Could you check a few things on this model? Use its own coordinates, in mm. A direction names the side the tool comes from. Coordinates: 2 decimals unless noted, no trailing zeros. Write each loop counter-clockwise with the first axis right and the second up, starting at its lowest first coordinate (ties: lowest second). Pieces come first, ordered by that corner, then holes.
Item 1: I want a section at A-A on x = 11. Please give me the cut outline in (y, z), then the cut area to 3 significant figures.
Item 2: I want a section at D-D on x = 23. Please give me the cut outline in (y, z).
Item 3: I want a section at B-B on y = -23. Please give me the cut outline in (x, z), then the cut area to 3 significant figures.
Item 4: Which directions (+Z, -Z, +X, -X, +Y, -Y) give clear straight access to the entire face, cutting with the end or side of a thin tool? Please do faces 4 (the cylindrical face through (-27.454, -13.85, 14.954)), 5 (the flat face through (34, 6, 15.5)), 6 (the flat face through (5, 4, 5.6)), 7 (the flat face through (23, -8, 25)).
Item 5: If I drill on probe 1 along Y at (x, z) = (27.5, 10.75); probe 2 along Y at (x, z) = (1, 19.5); probe 3 along Z at (x, y) = (5, 1), over which ranges is the centre line in solid material (lowest first)?
Item 6: For P1, Ø2, axis at y = 8.5, z = 21.5, coming from the -X side; P2, Ø4.5, axis at x = -30, z = 19.5, coming from the -Y side; P3, Ø0.6, axis at x = 29, z = 3, coming from the +Y side, each with a flat end and sliding along its axis, tell me the tip position at first contact or that it passes through.
Item 7: I want a section at C-C on y = -13.55. Please give me the cut outline in (x, z), then the cut area to 3 significant figures.
Item 8: Thinking about a two-plate mould opening in X: for faces 1 (the flat face through (29, -27.7, 4)), 2 (the flat face through (34, 6, 20.5)), 3 (the flat face through (30, -4, 20)), which applies, +X half, -X half, draft (parallel to the pull), parting line (faces both ways), or undercut?
from build123d import *

# Parameters (mm, degrees)
BOSS_EXTRUDE1_DEPTH = 25
SKETCH2_W           = 57.7
SKETCH2_H           = 16.5
CUT_EXTRUDE1_DEPTH  = 52.159456604
SKETCH3_W           = 30
SKETCH3_H           = 20
CUT_EXTRUDE2_DEPTH  = 7.5
CUT_EXTRUDE3_REACH  = 58.541
SKETCH4_R           = 2
SKETCH5_R           = 2
CUT_EXTRUDE4_DEPTH  = 1.5
SKETCH6_W           = 7
SKETCH6_H           = 8
BOSS_EXTRUDE2_DEPTH = 2
SKETCH7_W           = 4
SKETCH7_H           = 20.2
BOSS_EXTRUDE3_DEPTH = 2
BOSS_EXTRUDE4_DEPTH = 7
SKETCH9_W           = 32
SKETCH9_H           = 22
CUT_EXTRUDE5_DEPTH  = 2
FILLET1_R           = 1
FILLET2_R           = 1
SKETCH10_R          = 1
BOSS_EXTRUDE5_DEPTH = 1.5
FILLET3_R           = 1
BOSS_EXTRUDE6_DEPTH = 2.7
CUT_EXTRUDE6_REACH  = 82.092
SKETCH13_W          = 4.5
SKETCH13_H          = 8.8
BOSS_EXTRUDE7_DEPTH = 2
SKETCH14_W          = 10
SKETCH14_H          = 3.4
CUT_EXTRUDE7_DEPTH  = 54.232805215
SKETCH15_R          = 1.55
CUT_EXTRUDE8_DEPTH  = 2.5


with BuildPart() as part:
    # Sketch1 → Boss-Extrude1 (new body)
    with BuildSketch(Plane.XY):
        Polygon((0, 0), (30, 0), (30, -7.7), (-32.7, -7.7), (-32.7, -27.7), (35, -27.7), (35, 9), (0, 9), align=None)
    extrude(amount=BOSS_EXTRUDE1_DEPTH)

    # Sketch2 → Cut-Extrude1 (cut, through all)
    with BuildSketch(Plane.XY.offset(25)):
        with Locations((1.15, -19.45)):
            Rectangle(SKETCH2_W, SKETCH2_H)
    extrude(amount=-CUT_EXTRUDE1_DEPTH, mode=Mode.SUBTRACT)

    # Sketch3 → Cut-Extrude2 (cut)
    with BuildSketch(Plane(origin=(0, 9, 0), x_dir=(1, 0, 0), z_dir=(0, 1, 0))):
        with Locations((17.5, -12.5)):
            Rectangle(SKETCH3_W, SKETCH3_H)
    extrude(amount=-CUT_EXTRUDE2_DEPTH, mode=Mode.SUBTRACT)

    # Cut-Extrude3: up to this face of the body (flat: up to its plane)
    cut_extrude3_end = Plane(part.part.faces().sort_by_distance((17.5, 1.5, 12.5))[0])
    # Sketch4 → Cut-Extrude3 (cut, up to the picked face)
    with BuildSketch(Plane.XZ.offset(27.7), mode=Mode.PRIVATE) as cut_extrude3_sk1:
        with Locations(Location((30.5, 12.5, 0), (0, 0, 255.522487814))):
            Circle(SKETCH4_R)
    cut_extrude3_tool1 = split(extrude(cut_extrude3_sk1.sketch, amount=-CUT_EXTRUDE3_REACH, mode=Mode.PRIVATE), bisect_by=cut_extrude3_end, keep=Keep.BOTH, mode=Mode.PRIVATE)
    add(cut_extrude3_tool1.solids().sort_by(Axis((30.5, -27.7, 12.5), (0, 1, 0)))[0], mode=Mode.SUBTRACT)

    # Sketch5 → Cut-Extrude4 (cut)
    with BuildSketch(Plane(origin=(0, 1.5, 0), x_dir=(1, 0, 0), z_dir=(0, 1, 0))):
        with Locations(Location((5, -10, 0), (0, 0, 180))):
            Circle(SKETCH5_R)
    extrude(amount=-CUT_EXTRUDE4_DEPTH, mode=Mode.SUBTRACT)

    # Sketch6 → Boss-Extrude2 (add)
    with BuildSketch(Plane.XZ.offset(27.7)):
        with Locations((31.5, 21)):
            Rectangle(SKETCH6_W, SKETCH6_H)
        with Locations((31.5, 4)):
            Rectangle(SKETCH6_W, SKETCH6_H)
        with Locations((-29.2, 12.5)):
            Rectangle(SKETCH6_W, SKETCH6_H)
    extrude(amount=BOSS_EXTRUDE2_DEPTH)

    # Sketch7 → Boss-Extrude3 (add)
    with BuildSketch(Plane.XY.offset(25)):
        with Locations((2, -1.1)):
            Rectangle(SKETCH7_W, SKETCH7_H)
    extrude(amount=BOSS_EXTRUDE3_DEPTH)

    # Sketch8 → Boss-Extrude4 (add)
    with BuildSketch(Plane(origin=(35, 0, 0), x_dir=(0, 0, -1), z_dir=(1, 0, 0))):
        Polygon((0, -29.7), (-25, -33.360714286), (-25, -29.7), align=None)
    extrude(amount=-BOSS_EXTRUDE4_DEPTH)

    # Sketch9 → Cut-Extrude5 (cut)
    with BuildSketch(Plane(origin=(0, 9, 0), x_dir=(1, 0, 0), z_dir=(0, 1, 0))):
        with Locations((17.5, -12.5)):
            Rectangle(SKETCH9_W, SKETCH9_H)
    extrude(amount=-CUT_EXTRUDE5_DEPTH, mode=Mode.SUBTRACT)

    # Fillet1
    fillet1_edges = [part.edges().sort_by_distance(p)[0] for p in [
        (33.5, 8, 1.5),
        (33.5, 8, 23.5),
        (1.5, 8, 23.5),
        (1.5, 8, 1.5),
        (2.5, 4.25, 22.5),
        (2.5, 4.25, 2.5),
        (32.5, 4.25, 2.5),
        (32.5, 4.25, 22.5),
    ]]
    fillet(fillet1_edges, radius=FILLET1_R)

    # Fillet2
    fillet2_edges = [part.edges().sort_by_distance(p)[0] for p in [
        (4, -9.45, 25),
        (4, 4.5, 25),
        (0, -9.45, 25),
    ]]
    fillet(fillet2_edges, radius=FILLET2_R)
    fillet2_2_edges = [part.edges().sort_by_distance(p)[0] for p in [
        (20, 9, 25),
        (0, 9, 13.5),
        (17.5, 9, 0),
        (35, 9, 12.5),
        (28, -30.530357143, 25),
        (28, -28.7, 0),
        (28, -31.530357143, 12.5),
        (35, -31.530357143, 12.5),
        (-30.2, -27.7, 0),
        (-30.2, -27.7, 25),
        (-29.2, -29.7, 8.5),
        (-29.2, -29.7, 16.5),
        (-32.7, -28.7, 8.5),
        (-32.7, -28.7, 16.5),
        (-32.7, -27.7, 20.75),
        (-32.7, -29.7, 12.5),
        (-32.7, -27.7, 4.25),
        (-32.7, -7.7, 12.5),
        (-32.7, -17.7, 0),
        (-32.7, -17.7, 25),
        (35, -10.35, 0),
        (35, -12.180357143, 25),
        (0, -1.1, 27),
        (0, 4.5, 0),
        (4, -1.1, 27),
        (2, -11.2, 27),
        (2, 9, 27),
        (31.5, -33.360714286, 25),
        (31.5, -29.7, 0),
        (-25.7, -29.7, 12.5),
        (4.292893219, 9, 25.292893219),
    ]]
    fillet(fillet2_2_edges, radius=FILLET2_R - 0.0001)  # a hair under: the kernel refuses the full size

    # Sketch10 → Boss-Extrude5 (add)
    with BuildSketch(Plane(origin=(-27.7, 0, 0), x_dir=(0, 0, -1), z_dir=(1, 0, 0))):
        with Locations(Location((-14, -13.55, 0), (0, 0, 180))):
            Circle(SKETCH10_R)
        with Locations(Location((-11, -13.55, 0), (0, 0, 180))):
            Circle(SKETCH10_R)
    extrude(amount=BOSS_EXTRUDE5_DEPTH)

    # Fillet3
    fillet3_edges = [part.edges().sort_by_distance(p)[0] for p in [
        (-26.2, -13.55, 13),
        (-26.2, -13.55, 10),
    ]]
    fillet(fillet3_edges, radius=FILLET3_R)

    # Sketch11 → Boss-Extrude6 (add)
    with BuildSketch(Plane(origin=(0, 1.5, 0), x_dir=(1, 0, 0), z_dir=(0, 1, 0))):
        Polygon((2.5, -5.6), (2.5, -14.4), (7, -14.4), (7, -12.4), (3, -12.4), (3, -7.6), (7, -7.6), (7, -5.6), align=None)
    extrude(amount=BOSS_EXTRUDE6_DEPTH)

    # Cut-Extrude6: up to this face of the body (flat: up to its plane)
    cut_extrude6_end = Plane(part.part.faces().sort_by_distance((32.5, 4.25, 12.5))[0])
    # Sketch12 → Cut-Extrude6 (cut, up to the picked face)
    with BuildSketch(Plane(origin=(35, 0, 0), x_dir=(0, 0, -1), z_dir=(1, 0, 0)), mode=Mode.PRIVATE) as cut_extrude6_sk1:
        with BuildLine():
            Line((-20.5, 9), (-20.5, 4.5))
            ThreePointArc((-20.5, 4.5), (-18, 2), (-15.5, 4.5))
            Line((-15.5, 4.5), (-15.5, 9))
            Line((-15.5, 9), (-20.5, 9))
        make_face()
    cut_extrude6_tool1 = split(extrude(cut_extrude6_sk1.sketch, amount=-CUT_EXTRUDE6_REACH, mode=Mode.PRIVATE), bisect_by=cut_extrude6_end, keep=Keep.BOTH, mode=Mode.PRIVATE)
    add(cut_extrude6_tool1.solids().sort_by(Axis((35, 5.744167, 18), (-1, 0, 0)))[0], mode=Mode.SUBTRACT)

    # Sketch13 → Boss-Extrude7 (add)
    with BuildSketch(Plane(origin=(0, 4.2, 0), x_dir=(1, 0, 0), z_dir=(0, 1, 0))):
        with Locations((4.75, -10)):
            Rectangle(SKETCH13_W, SKETCH13_H)
    extrude(amount=BOSS_EXTRUDE7_DEPTH)

    # Sketch14 → Cut-Extrude7 (cut, through all)
    with BuildSketch(Plane(origin=(0, 0, 22.5), x_dir=(-1, 0, 0), z_dir=(0, 0, -1))):
        with Locations((-20, 3.2)):
            Rectangle(SKETCH14_W, SKETCH14_H)
    extrude(amount=-CUT_EXTRUDE7_DEPTH, mode=Mode.SUBTRACT)

    # Sketch15 → Cut-Extrude8 (cut)
    with BuildSketch(Plane.XY.offset(25)):
        with Locations((11, 3.2)):
            Circle(SKETCH15_R)
    extrude(amount=-CUT_EXTRUDE8_DEPTH, mode=Mode.SUBTRACT)


solid = part.part
Response values:
1. outline: (-11.2, 0) - (-7.7, 0) - (-7.7, 25) - (-11.2, 25) - close; (0, 0) - (8, 0) arc R1 ccw to (9, 1) - (9, 1.5) - (7, 1.5) - (7, 2.5) - (1.5, 2.5) - (1.5, 22.5) - (1.65, 22.5) - (1.65, 25) - (0, 25) - close; (4.75, 22.5) - (7, 22.5) - (7, 23.5) - (9, 23.5) - (9, 24) arc R1 ccw to (8, 25) - (4.75, 25) - close
1. area: 150 mm2
2. outline: (-11.2, 0) - (-7.7, 0) - (-7.7, 25) - (-11.2, 25) - close; (0, 0) - (8, 0) arc R1 ccw to (9, 1) - (9, 1.5) - (7, 1.5) - (7, 2.5) - (1.5, 2.5) - (1.5, 25) - (0, 25) - close; (4.9, 22.5) - (7, 22.5) - (7, 23.5) - (9, 23.5) - (9, 24) arc R1 ccw to (8, 25) - (4.9, 25) - close
3. outline: (-32.7, 1) arc R1 ccw to (-31.7, 0) - (-27.7, 0) - (-27.7, 25) - (-31.7, 25) arc R1 ccw to (-32.7, 24) - close; (30, 0) - (34, 0) arc R1 ccw to (35, 1) - (35, 24) arc R1 ccw to (34, 25) - (30, 25) - (30, 14.44) arc R2 cw (long way) to (30, 10.56) - close
3. area: 241 mm2
4. face 4: none
4. face 5: +X, +Y
4. face 6: +Y
4. face 7: +Z, +X, +Y, -Y
5. probe 1: y = -11.2 to -7.7, 0 to 1.5
5. probe 2: y = -11.2 to -7.7, 0 to 9
5. probe 3: z = 0 to 8, 12 to 25
6. P1: stops at x = 0
6. P2: stops at y = -27.7
6. P3: stops at y = 1.5
7. outline: (-32.7, 1) arc R1 ccw to (-31.7, 0) - (-27.7, 0) - (-27.7, 10) - (-27.2, 10) arc R1 ccw to (-27.2, 12) - (-27.7, 12) - (-27.7, 13) - (-27.2, 13) arc R1 ccw to (-27.2, 15) - (-27.7, 15) - (-27.7, 25) - (-31.7, 25) arc R1 ccw to (-32.7, 24) - close; (30, 0) - (34, 0) arc R1 ccw to (35, 1) - (35, 24) arc R1 ccw to (34, 25) - (30, 25) - (30, 14.44) arc R2 cw (long way) to (30, 10.56) - close
7. area: 246 mm2
8. face 1: undercut
8. face 2: draft
8. face 3: -X half
